For this review, take the finished solid that the model builds, in its own axes (mm). Face numbers are marked on the shaded views. A direction names the side the tool comes from. Round coordinates to 2 decimals unless told otherwise and drop trailing zeros. Order: outer loops, then holes, each group sorted by start corner. A loop starts at its lowest first (then second) coordinate and runs counter-clockwise, first axis right, second up. Notation, with made-up numbers: M 77.25,-20.5 L 124.25,-20.5 A13 cw 124.25,-0.5 Z; hole C 22.5,38 d6. An arc over 180 degrees is marked long. Put each result on its own line as item: value.
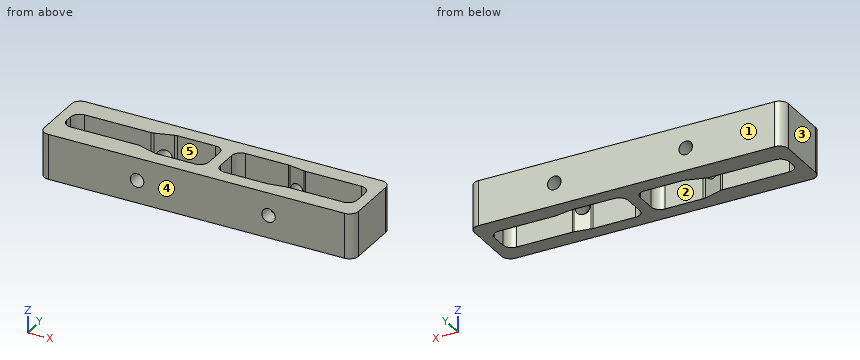
from build123d import *

# Parameters (mm, degrees)
F0_W     = 69.9
F0_H     = 15
F1_DEPTH = 5
F2_R     = 1.5
F3_DEPTH = 12.5
F4_R     = 2
F5_R     = 2


with BuildPart() as f1:
    # F0 (on Top) → F1 (new body, symmetric)
    with BuildSketch(Plane.XY):
        Rectangle(F0_W, F0_H)
        Polygon((-10.95, -4.15), (-15.45, -2.8), (-32.55, -2.8), (-32.55, 2.8), (-15.45, 2.8), (-10.95, 4.15), (-0.15, 4.15), (-0.15, -4.15), align=None, mode=Mode.SUBTRACT)
        Polygon((17.95, -3.65), (14.15, -4.3), (2.45, -4.3), (2.45, 4.3), (14.15, 4.3), (17.95, 3.65), (32.55, 3.65), (32.55, -3.65), align=None, mode=Mode.SUBTRACT)
    extrude(amount=F1_DEPTH, both=True)

    # F2 (on Front) → F3 (cut, symmetric)
    with BuildSketch(Plane.XZ):
        with Locations((-13.2, 0)):
            Circle(F2_R)
        with Locations((16.05, 0)):
            Circle(F2_R)
    extrude(amount=F3_DEPTH, both=True, mode=Mode.SUBTRACT)

    # F4
    f4_edges = [f1.edges().sort_by_distance(p)[0] for p in [
        (-34.95, 7.5, 0),
        (-34.95, -7.5, 0),
        (34.95, -7.5, 0),
        (34.95, 7.5, 0),
    ]]
    fillet(f4_edges, radius=F4_R)

    # F5
    f5_edges = [f1.edges().sort_by_distance(p)[0] for p in [
        (-32.55, 2.8, 0),
        (32.55, 3.65, 0),
        (32.55, -3.65, 0),
        (-32.55, -2.8, 0),
        (-15.45, 2.8, 0),
        (-10.95, 4.15, 0),
        (14.15, 4.3, 0),
        (17.95, 3.65, 0),
        (-15.45, -2.8, 0),
        (-10.95, -4.15, 0),
        (14.15, -4.3, 0),
        (17.95, -3.65, 0),
        (-0.15, 4.15, 0),
        (-0.15, -4.15, 0),
        (2.45, -4.3, 0),
        (2.45, 4.3, 0),
    ]]
    fillet(f5_edges, radius=F5_R)


solid = f1.part
(1) Draft analysis for pull direction X (two halves, no side actions). For the marked faces 3, 4 and 5, state which applies: released by +X, released by -X, zero draft, split by the parting line, or undercut.
A:
face 3: released by -X
face 4: zero draft
face 5: undercut
(2) For the marked faces 1 and 2, list the 3-axis set-ups (+Z, -Z, +X, -X, +Y, -Y) from which the entire face can be reached by the end or side of a thin tool; tool diameter is ignored.
A:
face 1: +Z, -Z, +X, -X, +Y
face 2: +Z, -Z
(3) Add section A-A on x = -18.5. Give the boundary of the cut face in (y, z), then the cut area to 3 significant figures.
A:
outline: M -7.5,-5 L -2.8,-5 L -2.8,5 L -7.5,5 Z; M 2.8,-5 L 7.5,-5 L 7.5,5 L 2.8,5 Z
area: 94.0 mm2
(4) Insertion check: pin 1 Ø4 at (x, z) = (16.05, 0) entering from -Y; pin 2 Ø2.5 at (x, z) = (-13.2, 0) entering from +Y. Each pin has a flat end and moves straight along its axis. Give the tip position at first contact, or say it passes through.
A:
pin 1: stops at y = -7.5
pin 2: passes through
(5) Add section B-B on x = 23. Give the boundary of the cut face in (y, z), then the cut area to 3 significant figures.
A:
outline: M -7.5,-5 L -3.65,-5 L -3.65,5 L -7.5,5 Z; M 3.65,-5 L 7.5,-5 L 7.5,5 L 3.65,5 Z
area: 77.0 mm2
(6) Add section C-C on z = -4. State how many separate pieces and enclosed holes the cut face has, then the cut area to 3 significant figures.
A:
separate pieces: 1
enclosed holes: 2
area: 598 mm2
(7) To check wall thickness, follow L1, parallel to X at y = 0.25, z = 2.25; L2, parallel to X at y = -4.7, z = 0; L3, parallel to Y at x = -21, z = 1.25. State the ranges of each line that lie inside material, in increasing order.
A:
L1: x = -34.95 to -32.55, -0.15 to 2.45, 32.55 to 34.95
L2: x = -34.95 to -14.7, -11.7 to 14.55, 17.55 to 34.95
L3: y = -7.5 to -2.8, 2.8 to 7.5
